The model under review builds one solid part; all positions refer to its coordinate system, in mm. A direction names the side the tool comes from. Coordinates: 2 decimals unless noted, no trailing zeros. Loops run counter-clockwise (first coordinate to the right, second up) from the corner with the lowest first, then second, coordinate; pieces in that order, holes last. Notation, with made-up numbers: (47.25, 43.5) - (66.25, 43.5) arc R33 cw to (66.25, 71.5) - close; hole circle Ø7 at (86, 82). An arc over 180 degrees is marked (long way). Answer in a Markdown table with one row per item. Add a question column.
(1) We need section D-D on z = -49.5. Write out the cut boundary in (x, y).
(2) We need section B-B on y = -69. Write out the cut boundary in (x, z).
(3) Mouldability with a two-part tool opening along Z and no side actions: class faces 4 (the flat face through (-21, -69, -26)), 5 (the cylindrical face through (15.195, -66.479, -61.487)), 6 (the flat face through (0, -69, -63)), 7 (the flat face through (-24, -69, 5)) as +Z half, -Z half, draft (parallel to the pull), parting line (faces both ways), or undercut.
(4) We need section A-A on x = -15. Write out the cut boundary in (y, z), plus the area to 3 significant figures.
(5) Machinability: for faces 1 (the flat face through (25.4, -68, -9.4)), 2 (the flat face through (0, -69, -57)), 3 (the flat face through (-13.6, -68, -61.4)), which of the approach directions +Z, -Z, +X, -X, +Y, -Y give a long, thin tool a straight path to every point of the face, cutting with its end or side? Answer none if there is none.
(6) For line 1 along X through (y, z) = (-70.25, -54); line 2 along Z through (x, y) = (24, -72.25); line 3 along Z through (x, y) = (15, -70.25), list the stretches that pass through material, from the lowest coordinate up.
(7) We need section C-C on z = -8. Give the number of separate pieces and of enclosed holes in the cut face, plus the area to 3 significant figures.
(8) For P1, Ø0.6, axis at x = -24.5, y = -68.5, coming from the -Z side; P2, Ø2.5, axis at x = -15, z = -60, coming from the -Y side; P3, Ø0.6, axis at y = -69, z = -61, coming from the +X side; P4, Ø1, axis at x = 18, y = -72.5, coming from the +Z side, all flat-tipped, find the tip position at first contact; note any pin that passes through.
from build123d import *

# Parameters (mm, degrees)
BOX905_W               = 6
BOX905_H               = 6
BOX905_DEPTH           = 2
BOX906_W               = 6
BOX906_H               = 6
BOX906_DEPTH           = 2
BOX907_W               = 6
BOX907_H               = 6
BOX907_DEPTH           = 2
BOX904_W               = 7
BOX904_H               = 6
BOX904_DEPTH           = 2
CYLINDER2651_R         = 1.5
CYLINDER2651_DEPTH     = 60
CYLINDER2652_R         = 1.5
CYLINDER2652_DEPTH     = 60
CYLINDER2653_R         = 1.5
CYLINDER2653_DEPTH     = 60
CYLINDER2650_R         = 1.5
CYLINDER2650_DEPTH     = 60
BOX894_W               = 42
BOX894_H               = 64
BOX894_DEPTH           = 50
BOX893_W               = 54
BOX893_H               = 68
BOX893_DEPTH           = 9
CHAMFER127_SIZE        = 3
CUT989_ROLL_ANGLE      = -90
CUT989_PLACEMENT_ANGLE = 180


with BuildPart() as krychle904:
    # Box905 → Box905 (new body)
    with BuildSketch(Plane(origin=(-18, 122, -48), x_dir=(1, 0, 0), z_dir=(0, 0, 1))):
        with Locations((3, 3)):
            Rectangle(BOX905_W, BOX905_H)
    extrude(amount=BOX905_DEPTH)


with BuildPart() as krychle905:
    # Box906 → Box906 (new body)
    with BuildSketch(Plane(origin=(21, 70, -48), x_dir=(1, 0, 0), z_dir=(0, 0, 1))):
        with Locations((3, 3)):
            Rectangle(BOX906_W, BOX906_H)
    extrude(amount=BOX906_DEPTH)


with BuildPart() as krychle906:
    # Box907 → Box907 (new body)
    with BuildSketch(Plane(origin=(12, 122, -48), x_dir=(1, 0, 0), z_dir=(0, 0, 1))):
        with Locations((3, 3)):
            Rectangle(BOX907_W, BOX907_H)
    extrude(amount=BOX907_DEPTH)


with BuildPart() as compound1179:
    # Box904 → Box904 (new body)
    with BuildSketch(Plane(origin=(-28, 70, -48), x_dir=(1, 0, 0), z_dir=(0, 0, 1))):
        with Locations((3.5, 3)):
            Rectangle(BOX904_W, BOX904_H)
    extrude(amount=BOX904_DEPTH)

    # Compound1179: union Krychle904, Krychle905, Krychle906
    add(krychle904.part)
    add(krychle905.part)
    add(krychle906.part)


with BuildPart() as compound1179_1:
    # Compound1179 placement: moved
    add(compound1179.part.moved(Location((0, 0, 118))))


with BuildPart() as obj1:
    # Cylinder2651 → Cylinder2651 (new body)
    with BuildSketch(Plane(origin=(-24, 73, -80), x_dir=(1, 0, 0), z_dir=(0, 0, 1))):
        Circle(CYLINDER2651_R)
    extrude(amount=CYLINDER2651_DEPTH)


with BuildPart() as obj2:
    # Cylinder2652 → Cylinder2652 (new body)
    with BuildSketch(Plane(origin=(-15, 125, -80), x_dir=(1, 0, 0), z_dir=(0, 0, 1))):
        Circle(CYLINDER2652_R)
    extrude(amount=CYLINDER2652_DEPTH)


with BuildPart() as obj3:
    # Cylinder2653 → Cylinder2653 (new body)
    with BuildSketch(Plane(origin=(15, 125, -80), x_dir=(1, 0, 0), z_dir=(0, 0, 1))):
        Circle(CYLINDER2653_R)
    extrude(amount=CYLINDER2653_DEPTH)


with BuildPart() as compound1172:
    # Cylinder2650 → Cylinder2650 (new body)
    with BuildSketch(Plane(origin=(24, 73, -80), x_dir=(1, 0, 0), z_dir=(0, 0, 1))):
        Circle(CYLINDER2650_R)
    extrude(amount=CYLINDER2650_DEPTH)

    # Compound1172: union obj1, obj2, obj3
    add(obj1.part)
    add(obj2.part)
    add(obj3.part)


with BuildPart() as compound1172_1:
    # Compound1172 placement: moved
    add(compound1172.part.moved(Location((0, 0, 120))))


with BuildPart() as krychle893:
    # Box894 → Box894 (new body)
    with BuildSketch(Plane(origin=(-21, 58, 40), x_dir=(1, 0, 0), z_dir=(0, 0, 1))):
        with Locations((21, 32)):
            Rectangle(BOX894_W, BOX894_H)
    extrude(amount=BOX894_DEPTH)


with BuildPart() as cut989:
    # Box893 → Box893 (new body)
    with BuildSketch(Plane(origin=(-27, 60, 76), x_dir=(1, 0, 0), z_dir=(0, 0, 1))):
        with Locations((27, 34)):
            Rectangle(BOX893_W, BOX893_H)
    extrude(amount=BOX893_DEPTH)

    # Cut978: cut Krychle893
    add(krychle893.part, mode=Mode.SUBTRACT)


with BuildPart() as cut989_1:
    # Cut978 placement: moved
    add(cut989.part.moved(Location((0, 0, -9))))

    # Chamfer127
    chamfer127_edges = [cut989_1.edges().sort_by_distance(p)[0] for p in [
        (-27, 128, 71.5),
        (27, 128, 71.5),
    ]]
    chamfer(chamfer127_edges, length=CHAMFER127_SIZE)

    # Cut979: cut Compound1172
    add(compound1172_1.part, mode=Mode.SUBTRACT)

    # Cut989: cut Compound1179
    add(compound1179_1.part, mode=Mode.SUBTRACT)


with BuildPart() as cut989_2:
    # Cut989 roll: moved
    add(cut989_1.part.rotate(Axis((0, 0, 0), (1, 0, 0)), CUT989_ROLL_ANGLE))


with BuildPart() as cut989_3:
    # Cut989 placement: moved
    add(cut989_2.part.moved(Location((0, 2, 65))).rotate(Axis((0, 2, 65), (0, 0, 1)), CUT989_PLACEMENT_ANGLE))


solid = cut989_3.part
Outcome:
| question | item | result |
|---|---|---|
| 1 | outline | (-27, -74) - (-21, -74) - (-21, -65) - (-27, -65) - close; (21, -74) - (27, -74) - (27, -65) - (21, -65) - close |
| 2 | outline | (-27, -60) - (-24, -63) - (-18, -63) - (-18, -57) - (-21, -57) - (-21, -11) - (-27, -11) - close; (-27, -5) - (-21, -5) - (-21, 5) - (-27, 5) - close; (-12, -63) - (12, -63) - (12, -57) - (-12, -57) - close; (18, -63) - (24, -63) - (27, -60) - (27, -11) - (21, -11) - (21, -57) - (18, -57) - close; (21, -5) - (27, -5) - (27, 5) - (21, 5) - close |
| 3 | face 4 | draft |
| 3 | face 5 | undercut |
| 3 | face 6 | -Z half |
| 3 | face 7 | +Z half |
| 4 | outline | (-74, -63) - (-70, -63) - (-70, -61.5) - (-74, -61.5) - close; (-74, -58.5) - (-70, -58.5) - (-70, -57) - (-74, -57) - close; (-68, -63) - (-65, -63) - (-65, -61.5) - (-68, -61.5) - close; (-68, -58.5) - (-65, -58.5) - (-65, -57) - (-68, -57) - close |
| 4 | area | 21.0 mm² |
| 5 | face 1 | +X, -X |
| 5 | face 2 | +Z, +Y, -Y |
| 5 | face 3 | +Z, -Z |
| 6 | line 1 | -27 to -21, 21 to 27 |
| 6 | line 2 | -63 to -9.5, -6.5 to 5 |
| 6 | line 3 | -63 to -61.5, -58.5 to -57 |
| 7 | separate pieces | 8 |
| 7 | enclosed holes | 0 |
| 7 | area | 42.0 mm² |
| 8 | P1 | z = -62.8 |
| 8 | P2 | through |
| 8 | P3 | x = 26.3 |
| 8 | P4 | z = -57 |
